from build123d import *

# Parameters (mm, degrees)
BOSS_EXTRUDE2_DEPTH = 3


with BuildPart() as part:
    # Sketch1 → Boss-Extrude2 (new body)
    with BuildSketch(Plane(origin=(0, 0, 0), x_dir=(1, 0, 0), z_dir=(0, 1, 0))):
        with BuildLine():
            Line((0, 0), (-3.8, 0))
            ThreePointArc((-3.8, 0), (-5.3, 1.5), (-3.8, 3))
            Line((-3.8, 3), (13.04, 3))
            Line((13.04, 3), (12.868254879, 4.963055716))
            ThreePointArc((12.868254879, 4.963055716), (12.228877244, 6.545570894), (10.813877905, 7.5))
            Line((10.813877905, 7.5), (6.156299709, 8.923964556))
            ThreePointArc((6.156299709, 8.923964556), (5.230638373, 9.525590656), (4.765198448, 10.526674344))
            ThreePointArc((4.765198448, 10.526674344), (-0.630284052, 14.79), (-5.3, 9.742136094))
            Line((-5.3, 9.742136094), (-5.3, 7.77))
            Line((-5.3, 7.77), (-7.99, 7.77))
            ThreePointArc((-7.99, 7.77), (-14.26, 1.5), (-7.99, -4.77))
            Line((-7.99, -4.77), (-1.5, -4.77))
            ThreePointArc((-1.5, -4.77), (-0.439339828, -4.330660172), (0, -3.27))
            Line((0, -3.27), (0, 0))
        make_face()
    extrude(amount=BOSS_EXTRUDE2_DEPTH)


solid = part.part
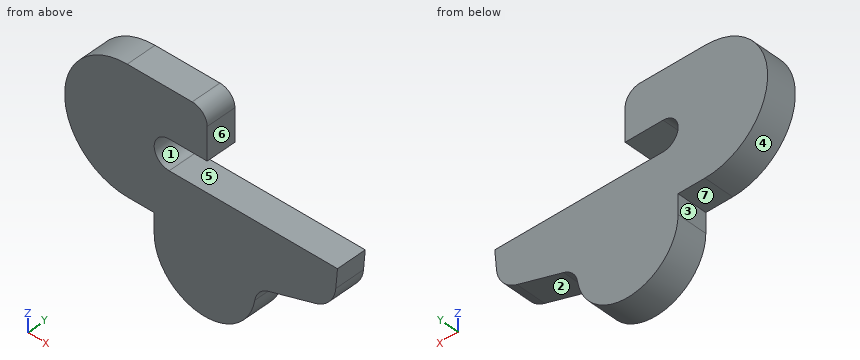
Geometry: final body of the model. Coordinates: model frame, mm. Face numbers are marked on the shaded views. A direction names the side the tool comes from. Give positions to 0.01 mm unless a question says otherwise; leave off trailing zeros. Loops run counter-clockwise (first coordinate to the right, second up) from the corner with the lowest first, then second, coordinate; pieces in that order, holes last. Notation, with made-up numbers: (28, 13.25) - (40, 13.25) arc R31 cw to (40, 47.25) - close; hole circle Ø8 at (42.25, 35). An arc over 180 degrees is marked (long way). Answer as CSV lines item,"result". Start each with the question number.
1. Reachability of the marked faces 4, 5, 6 and 7 from +Z, -Z, +X, -X, +Y, -Y: full face, straight path, thin tool, end or side. Return the list, or none.
2. Ray query, L1, parallel to Z at x = -4.5, y = 0.7; L2, parallel to Z at x = -1.25, y = 1.25; L3, parallel to Z at x = -7.25, y = 1.95. Return the intervals inside material, ascending.
3. Section C-C, the plane z = -1.5. Return loops of the section in (x, y).
4. Pin query (flat end, axial travel): P1, Ø0.9, axis at x = 8.5, y = 1.5, coming from the +Z side; P2, Ø4, axis at x = -8, z = -12.5, coming from the +Y side (3 decimals); P3, Ø0.8, axis at x = -7, y = 1, coming from the -Z side. Return the tip coordinate at first contact, or that it passes through.
5. Section A-A, the plane y = 0.6. Return loops of the section in (x, z).
6. Draft query along Z for the marked faces 1, 2 and 3. Return one class per face: released by +Z, released by -Z, zero draft, split by the parting line, or undercut.
7. Section B-B, the plane x = 7.75. Return loops of the section in (y, z), plus the area to 3 significant figures.
Answers:
1,face 4,"-X, +Y, -Y"
1,face 5,"+X, +Y, -Y"
1,face 6,"+Z, +X, +Y, -Y"
1,face 7,"-Z, -X, +Y, -Y"
2,L1,"z = -12.47 to -2.83, -0.17 to 4.77"
2,L2,"z = -14.7 to -3, 0 to 4.75"
2,L3,"z = -7.77 to 4.77"
3,outline,"(-14.26, 0) - (-5.3, 0) - (-5.3, 3) - (-14.26, 3) - close"
4,P1,"stops at z = -3"
4,P2,"passes through"
4,P3,"stops at z = -7.77"
5,outline,"(-7.99, -7.77) - (-5.3, -7.77) - (-5.3, -9.74) arc R5.06 ccw to (4.77, -10.53) arc R2 cw to (6.16, -8.92) - (10.81, -7.5) arc R2.92 ccw to (12.87, -4.96) - (13.04, -3) - (-3.8, -3) arc R1.5 cw to (-3.8, 0) - (0, 0) - (0, 3.27) arc R1.5 ccw to (-1.5, 4.77) - (-7.99, 4.77) arc R6.27 ccw to start"
6,face 1,"undercut"
6,face 2,"released by -Z"
6,face 3,"zero draft"
7,outline,"(0, -8.44) - (3, -8.44) - (3, -3) - (0, -3) - close"
7,area,"16.3 mm2"
